from build123d import *

# Parameters (mm, degrees)
CROQUIS2_W              = 140
CROQUIS2_H              = 70
SALIENTE_EXTRUIR1_DEPTH = 3
CROQUIS3_R              = 1.5
CORTAR_EXTRUIR1_DEPTH   = 3
CHAFL_N2_SIZE           = 15
CROQUIS4_R              = 1.5
CROQUIS4_W              = 3
CROQUIS4_H              = 38.326321521
CROQUIS4_W_2            = 30
CROQUIS4_H_2            = 3
CROQUIS4_W_3            = 5
CROQUIS4_H_3            = 45
CORTAR_EXTRUIR2_DEPTH   = 3


with BuildPart() as part:
    # Croquis2 → Saliente-Extruir1 (new body)
    with BuildSketch(Plane.XY):
        Rectangle(CROQUIS2_W, CROQUIS2_H)
    extrude(amount=SALIENTE_EXTRUIR1_DEPTH)

    # Croquis3 → Cortar-Extruir1 (cut)
    with BuildSketch(Plane.XY.offset(3)):
        with Locations((-65, -30)):
            Circle(CROQUIS3_R)
        with Locations((65, -30)):
            Circle(CROQUIS3_R)
        with Locations((0, -30)):
            Circle(CROQUIS3_R)
        with Locations((-60, 25)):
            Circle(CROQUIS3_R)
        with Locations((60, 25)):
            Circle(CROQUIS3_R)
        with Locations((0, 25)):
            Circle(CROQUIS3_R)
    extrude(amount=-CORTAR_EXTRUIR1_DEPTH, mode=Mode.SUBTRACT)

    # Chaflán2
    chafl_n2_edges = [part.edges().sort_by_distance(p)[0] for p in [
        (-70, 35, 1.5),
        (70, 35, 1.5),
    ]]
    chamfer(chafl_n2_edges, length=CHAFL_N2_SIZE)

    # Croquis4 → Cortar-Extruir2 (cut)
    with BuildSketch(Plane.XY.offset(3)):
        with Locations((-16.783900612, 23.326321521)):
            Circle(CROQUIS4_R)
        with Locations((16.216099388, 23.326321521)):
            Circle(CROQUIS4_R)
        with Locations((-16.783900612, -30)):
            Circle(CROQUIS4_R)
        with Locations((16.216099388, -30)):
            Circle(CROQUIS4_R)
        with Locations((13, -5.836839239)):
            Rectangle(CROQUIS4_W, CROQUIS4_H)
        with Locations((-13, -5.836839239)):
            Rectangle(CROQUIS4_W, CROQUIS4_H)
        with Locations((42.309397606, -30)):
            Rectangle(CROQUIS4_W_2, CROQUIS4_H_2)
        with Locations((-62.5, -3.320076901)):
            Rectangle(CROQUIS4_W_3, CROQUIS4_H_3)
    extrude(amount=-CORTAR_EXTRUIR2_DEPTH, mode=Mode.SUBTRACT)


solid = part.part
The model under review builds one solid part; all positions refer to its coordinate system, in mm. A direction names the side the tool comes from. Round coordinates to 2 decimals unless told otherwise and drop trailing zeros. Loops run counter-clockwise (first coordinate to the right, second up) from the corner with the lowest first, then second, coordinate; pieces in that order, holes last. Notation, with made-up numbers: (-20, -22) - (27, -22) arc R17 cw to (27, 7) - close; hole circle Ø8 at (-17.5, 24.5). An arc over 180 degrees is marked (long way). Use CSV: the item, a comma, the result in double quotes.
(1) Take a section at D-D, the plane y = 1. Give the boundary of the cut face in (x, z), plus the area to 3 significant figures.
Working result:
outline,"(-70, 0) - (-65, 0) - (-65, 3) - (-70, 3) - close; (-60, 0) - (-14.5, 0) - (-14.5, 3) - (-60, 3) - close; (-11.5, 0) - (11.5, 0) - (11.5, 3) - (-11.5, 3) - close; (14.5, 0) - (70, 0) - (70, 3) - (14.5, 3) - close"
area,"387 mm^2"
(2) Take a section at C-C, the plane x = 0. Give the boundary of the cut face in (y, z).
Working result:
outline,"(-35, 0) - (-31.5, 0) - (-31.5, 3) - (-35, 3) - close; (-28.5, 0) - (23.5, 0) - (23.5, 3) - (-28.5, 3) - close; (26.5, 0) - (35, 0) - (35, 3) - (26.5, 3) - close"
(3) Clearance check with a flat-ended pin moving along its axis: P1, Ø2.5, axis at x = -60, y = 25, coming from the -Z side. State where the tip first meets the part, or that it passes through.
Working result:
P1,"passes through"
(4) The part is to be moulded in two halves that separate along X. For faces 1 (the flat face through (63, 27, 1)), 2 (the flat face through (27.309, -30, 2)), 3 (the flat face through (-1, 0, 3)), say which applies: pulls with the +X half, pulls with the -X half, needs draft (parallel to the pull), parting line crosses it, or undercut.
Working result:
face 1,"pulls with the +X half"
face 2,"undercut"
face 3,"needs draft"
(5) For line 1 (X direction, y = 12, z = 0.3); line 2 (X direction, y = 16, z = 2.8); line 3 (Y direction, x = 42.5, z = 0.55), list the stretches that pass through material, from the lowest coordinate up.
Working result:
line 1,"x = -70 to -65, -60 to -14.5, -11.5 to 11.5, 14.5 to 70"
line 2,"x = -70 to -65, -60 to 70"
line 3,"y = -35 to -31.5, -28.5 to 35"
(6) Machinability: for faces 4 (the flat face through (70, -8, 1)), 5 (the flat face through (-13, -25, 2)), which of the approach directions +Z, -Z, +X, -X, +Y, -Y give a long, thin tool a straight path to every point of the face, cutting with its end or side? Answer none if there is none.
Working result:
face 4,"+Z, -Z, +X, +Y, -Y"
face 5,"+Z, -Z"
(7) Take a section at A-A, the plane x = 65. Give the boundary of the cut face in (y, z).
Working result:
outline,"(-35, 0) - (-31.5, 0) - (-31.5, 3) - (-35, 3) - close; (-28.5, 0) - (25, 0) - (25, 3) - (-28.5, 3) - close"
(8) Take a section at B-B, the plane y = 16.5. Give the boundary of the cut face in (x, z), plus the area to 3 significant figures.
Working result:
outline,"(-70, 0) - (-65, 0) - (-65, 3) - (-70, 3) - close; (-60, 0) - (70, 0) - (70, 3) - (-60, 3) - close"
area,"405 mm^2"
